Solid Edge part; units mm, degrees
sketch "Sketch1" plane through (60.3162, 60.3162, 0) normal (0, 0, 1) x (1, 0, 0)
  circle A0 centre (-60.3162, -60.3162) radius 43.7
extrude "Protrusion1" add sketch "Sketch1" along normal blind 30
hole "Bohrung_1" at (-30, 0, 30) direction (0, 0, -1) diameter 3.242 depth 13 thread major 4 thread length 8
pattern_circular "Pattern1" count 8 over 360 about axis through (0, 0, 30) along (0, 0, -1) of "Bohrung_1"
sketch "Sketch2" plane through (0, 0, 30) normal (0, 0, 1) x (0, 1, 0)
  circle A0 centre (0, 0) radius 12.5
extrude "Cutout1" cut sketch "Sketch2" against normal up to next
hole "Bohrung_2" at (-11.4805, 27.7164, 30) direction (0, 0, -1) diameter 3.242 depth 12 counterbore diameter 8 counterbore depth 3 thread major 4 thread length 10
pattern_circular "Pattern3" count 8 over 360 about axis through (0, 0, 30) along (0, 0, 1) of "Bohrung_2"
chamfer "Fase_1" distance 1 angle 45 1 edges at (-43.7, 0, 30)
Verification items for the finished model (mm, model axes). Coordinates: 2 decimals unless noted, no trailing zeros. Write each loop counter-clockwise with the first axis right and the second up, starting at its lowest first coordinate (ties: lowest second). Pieces come first, ordered by that corner, then holes. Notation, with made-up numbers: (22, 8) - (32, 8) arc R22 cw to (32, 33) - close; hole circle Ø10 at (1.5, -22.5). An arc over 180 degrees is marked (long way). One line per question, with ' | ' between items. Start each with the question number.
1. Section check A-A (x = 0). Enter the section's corners in (y, z).
2. Material ranges on line 1 along Y through (x, z) = (0, 24.25); line 2 along X through (y, z) = (-20.5, 26); line 3 along Z through (x, y) = (12, -26), recorded low to high.
3. Gauge pin test, flat ends, axial feed: P1, Ø6.5, axis at x = -27.72, y = -11.48, coming from the +Z side; P2, Ø3, axis at y = -7, z = 15, coming from the +X side; P3, Ø2.5, axis at x = 11.5, y = -27.5, coming from the +Z side. Record the tip position at first contact, or that the pin passes through.
4. Section check C-C (z = 24). Count the separate pieces of the cut face and the enclosed holes in it, plus the area to 3 significant figures.
5. Draft check along X on faces 1 (the cylindrical face through (-9.47, 42.66, 14.3)), 2 (the flat face through (26, 12, 27)), 3 (the cylindrical face through (26.845, 12.847, 22.437)). Enter one of: released by +X, released by -X, zero draft, split by the parting line, or undercut.
Computed values:
1) outline: (-43.7, 0) - (-12.5, 0) - (-12.5, 30) - (-28.38, 30) - (-28.38, 17) - (-31.62, 17) - (-31.62, 30) - (-42.7, 30) - (-43.7, 29) - close; (12.5, 0) - (43.7, 0) - (43.7, 29) - (42.7, 30) - (31.62, 30) - (31.62, 17) - (28.38, 17) - (28.38, 30) - (12.5, 30) - close
2) line 1: -43.7 to -31.62, -28.38 to -12.5, 12.5 to 28.38, 31.62 to 43.7 | line 2: -38.59 to -22.67, -19.76 to 19.76, 22.67 to 38.59 | line 3: 0 to 27
3) P1: z = 27 | P2: x = 43.35 | P3: z = 18
4) separate pieces: 1 | enclosed holes: 17 | area: 5,380 mm²
5) face 1: split by the parting line | face 2: undercut | face 3: undercut
